from build123d import *

# Parameters (mm, degrees)
SKETCH1_W           = 50
SKETCH1_H           = 50
SKETCH1_R           = 8
SKETCH1_R_2         = 1.5
BOSS_EXTRUDE1_DEPTH = 9.7
FILLET2_R           = 10
BOSS_EXTRUDE3_DEPTH = 5
CIRPATTERN6_COUNT   = 2
CUT_EXTRUDE1_DEPTH  = 2.5
FILLET3_R           = 4
CHAMFER2_SIZE       = 5


with BuildPart() as part:
    # Sketch1 → Boss-Extrude1 (new body)
    with BuildSketch(Plane.XY):
        Rectangle(SKETCH1_W, SKETCH1_H)
        Circle(SKETCH1_R, mode=Mode.SUBTRACT)
        with Locations((16.6, 0)):
            Circle(SKETCH1_R_2, mode=Mode.SUBTRACT)
        with Locations((0, -16.6)):
            Circle(SKETCH1_R_2, mode=Mode.SUBTRACT)
        with Locations((-16.6, 0)):
            Circle(SKETCH1_R_2, mode=Mode.SUBTRACT)
        with Locations((0, 16.6)):
            Circle(SKETCH1_R_2, mode=Mode.SUBTRACT)
    extrude(amount=BOSS_EXTRUDE1_DEPTH)

    # Fillet2
    fillet2_edges = [part.edges().sort_by_distance(p)[0] for p in [
        (-25, -25, 4.85),
        (-25, 25, 4.85),
        (25, 25, 4.85),
        (25, -25, 4.85),
    ]]
    fillet(fillet2_edges, radius=FILLET2_R)

    # Sketch7 → Boss-Extrude3 (add)
    with BuildSketch(Plane(origin=(25, 0, 0), x_dir=(0, 0, -1), z_dir=(1, 0, 0))):
        with BuildLine():
            Line((25.4, 5), (0, 5))
            Line((0, 5), (0, 2.6))
            Line((0, 2.6), (17.4, 2.6))
            ThreePointArc((17.4, 2.6), (19.238477631, 1.838477631), (20, 0))
            ThreePointArc((20, 0), (19.238477631, -1.838477631), (17.4, -2.6))
            Line((17.4, -2.6), (0, -2.6))
            Line((0, -2.6), (0, -5))
            Line((0, -5), (25.4, -5))
            Line((25.4, -5), (25.4, 5))
        make_face()
        Polygon((0, 5), (-9.7, 5), (-9.7, -5), (0, -5), (0, -2.6), (0, 2.6), align=None)
    boss_extrude3 = extrude(amount=BOSS_EXTRUDE3_DEPTH)

    # CirPattern6: Boss-Extrude3 ×2 about axis
    cirpattern6_axis = Axis((0, 0, 0), (0, 0, 1))
    for i in range(1, CIRPATTERN6_COUNT):
        add(boss_extrude3.rotate(cirpattern6_axis, i * 360 / CIRPATTERN6_COUNT))

    # Sketch9 → Cut-Extrude1 (cut)
    with BuildSketch(Plane(origin=(0, 0, 0), x_dir=(-1, 0, 0), z_dir=(0, 0, -1))):
        Polygon((2.801592181, -15.132762794), (2.801592181, -18.257762794), (0.095262794, -19.820262794), (-2.611066592, -18.257762794), (-2.611066592, -15.132762794), (0.095262794, -13.570262794), align=None)
        Polygon((18.1625, -2.706329387), (15.0375, -2.706329387), (13.475, 0), (15.0375, 2.706329387), (18.1625, 2.706329387), (19.725, 0), align=None)
        Polygon((2.611066592, 14.942237206), (-0.095262794, 13.379737206), (-2.801592181, 14.942237206), (-2.801592181, 18.067237206), (-0.095262794, 19.629737206), (2.611066592, 18.067237206), align=None)
        Polygon((-13.475, -0.190525589), (-15.0375, -2.896854976), (-18.1625, -2.896854976), (-19.725, -0.190525589), (-18.1625, 2.515803798), (-15.0375, 2.515803798), align=None)
    extrude(amount=-CUT_EXTRUDE1_DEPTH, mode=Mode.SUBTRACT)

    # Fillet3
    fillet3_edges = [part.edges().sort_by_distance(p)[0] for p in [
        (27.5, -5, -25.4),
        (27.5, 5, -25.4),
        (-27.5, 5, -25.4),
        (-27.5, -5, -25.4),
    ]]
    fillet(fillet3_edges, radius=FILLET3_R)

    # Chamfer2
    # the kernel refuses this chamfer: 5 mm, written as the material it adds along each edge
    with BuildSketch(Plane(origin=(-25, 5, 0), x_dir=(-0.9996219169112968, -0.027495876610586147, 0), z_dir=(0, 0, 1)), Plane(origin=(25, 5, 0), x_dir=(-0.027495876610586317, 0.9996219169112968, 0), z_dir=(0, 0, 1))) as chamfer2_piece_1:
        Polygon((CHAMFER2_SIZE * 0.999621916911, -CHAMFER2_SIZE * 0.0274958766106), (-CHAMFER2_SIZE * 0.0274958766106, -CHAMFER2_SIZE * 0.999621916911), (0, 0), align=None)
    extrude(amount=9.7)
    with BuildSketch(Plane(origin=(-25, -5, 0), x_dir=(-0.9996219169112968, 0.02749587661058649, 0), z_dir=(0, 0, 1)), Plane(origin=(25, -5, 0), x_dir=(-0.027495876610586317, -0.9996219169112968, 0), z_dir=(0, 0, 1))) as chamfer2_piece_2:
        Polygon((CHAMFER2_SIZE * 0.999621916911, CHAMFER2_SIZE * 0.0274958766106), (-CHAMFER2_SIZE * 0.0274958766106, CHAMFER2_SIZE * 0.999621916911), (0, 0), align=None)
    extrude(amount=9.7)


solid = part.part
Verification items for the finished model (mm, model axes). A direction names the side the tool comes from. Round coordinates to 2 decimals unless told otherwise and drop trailing zeros. Loops run counter-clockwise (first coordinate to the right, second up) from the corner with the lowest first, then second, coordinate; pieces in that order, holes last. Notation, with made-up numbers: (1, 89) - (45, 89) arc R27 ccw to (45, 124) - close; hole circle Ø11 at (2, 46). An arc over 180 degrees is marked (long way). Write item = value, one per line.
Q1. Depth check by flat-ended pin: pin 1 (2.5 mm diameter, centred on x = 0, y = 16.6, fed in from -Z); pin 2 (2.5 mm diameter, centred on x = 28.5, z = -9.5, fed in from +Y); pin 3 (0.8 mm diameter, centred on x = 16, z = 1, fed in from -Y); pin 4 (4.5 mm diameter, centred on x = 0, y = -18, fed in from -Z). Enter the tip coordinate at first touch or a pass-through.
Here are the results:
pin_1 = through
pin_2 = 5
pin_3 = -24.98
pin_4 = 0
Q2. Mould release check, pull along Y, two halves, no side actions. Record for faces 4 (the flat face through (0, 25, 5)), 5 (the flat face through (-25, 12, 5)), 6 (the flat face through (1.43, 14.15, 1.23)): +Y half, -Y half, draft (parallel to the pull), parting line (faces both ways), or undercut.
Here are the results:
face_4 = +Y half
face_5 = draft
face_6 = undercut
Q3. Material ranges on L1, parallel to Y at x = 0, z = 6.5; L2, parallel to Y at x = 27, z = -6; L3, parallel to Y at x = -0.5, z = 7, recorded low to high.
Here are the results:
L1 = -25 to -18.1, -15.1 to -8, 8 to 15.1, 18.1 to 25
L2 = -5 to -2.6, 2.6 to 5
L3 = -25 to -18.01, -15.19 to -7.98, 7.98 to 15.19, 18.01 to 25
Q4. Sectioned sample at A-A on z = 4.5. Record the boundary of the cut face in (x, y).
Here are the results:
outline = (-30, -5) - (-25, -10) - (-25, -15) arc R10 ccw to (-15, -25) - (15, -25) arc R10 ccw to (25, -15) - (25, -10) - (30, -5) - (30, 5) - (25, 10) - (25, 15) arc R10 ccw to (15, 25) - (-15, 25) arc R10 ccw to (-25, 15) - (-25, 10) - (-30, 5) - close; hole circle Ø3 at (-16.6, 0); hole circle Ø16 at (0, 0); hole circle Ø3 at (0, -16.6); hole circle Ø3 at (0, 16.6); hole circle Ø3 at (16.6, 0)
Q5. Sectioned sample at B-B on z = -7. Record the boundary of the cut face in (x, y).
Here are the results:
outline = (-30, -5) - (-25, -5) - (-25, -2.6) - (-30, -2.6) - close; (-30, 2.6) - (-25, 2.6) - (-25, 5) - (-30, 5) - close; (25, -5) - (30, -5) - (30, -2.6) - (25, -2.6) - close; (25, 2.6) - (30, 2.6) - (30, 5) - (25, 5) - close
Q6. Tool access check on faces 1 (the cylindrical face through (27.535, 3.859, -24.197)), 2 (the flat face through (-27, -5, -11)), 3 (the flat face through (-18, 1, 2.5)). Record the directions out of +Z, -Z, +X, -X, +Y, -Y that give a thin tool (end or side, any length) a straight path to the whole face; none if there is none.
Here are the results:
face_1 = -Z, +X, -X, +Y
face_2 = -Z, +X, -X, -Y
face_3 = -Z
Q7. Sectioned sample at C-C on x = -5.5. Record the boundary of the cut face in (y, z), plus the area to 3 significant figures.
Here are the results:
outline = (-25, 0) - (-5.81, 0) - (-5.81, 9.7) - (-25, 9.7) - close; (5.81, 0) - (25, 0) - (25, 9.7) - (5.81, 9.7) - close
area = 372 mm^2
Q8. Sectioned sample at D-D on y = -16.6. Record the boundary of the cut face in (x, z).
Here are the results:
outline = (-24.87, 0) - (-2.8, 0) - (-2.8, 2.5) - (-1.5, 2.5) - (-1.5, 9.7) - (-24.87, 9.7) - close; (1.5, 2.5) - (2.61, 2.5) - (2.61, 0) - (24.87, 0) - (24.87, 9.7) - (1.5, 9.7) - close
